```python
from build123d import *

# Parameters (mm, degrees)
F0_R     = 4.8825627193
F0_R_2   = 12.5
F1_DEPTH = 20
F2_R     = 5


with BuildPart() as f1:
    # F0 (on Front) → F1 (new body)
    with BuildSketch(Plane.XZ):
        with BuildLine():
            Line((-24.8438301682, -42.8251363337), (24.8438301682, -42.8251363337))
            Line((24.8438301682, -42.8251363337), (44.8438301682, -20.8251363337))
            Line((44.8438301682, -20.8251363337), (44.8438301682, 42.8251363337))
            Line((44.8438301682, 42.8251363337), (19.4535404444, 42.8251363337))
            Line((19.4535404444, 42.8251363337), (19.4535404444, 22.1680208296))
            ThreePointArc((19.4535404444, 22.1680208296), (17.9890743503, 18.6324869236), (14.4535404444, 17.1680208296))
            Line((14.4535404444, 17.1680208296), (-14.4535404444, 17.1680208296))
            ThreePointArc((-14.4535404444, 17.1680208296), (-17.9890743503, 18.6324869236), (-19.4535404444, 22.1680208296))
            Line((-19.4535404444, 22.1680208296), (-19.4535404444, 42.8251363337))
            Line((-19.4535404444, 42.8251363337), (-44.8438301682, 42.8251363337))
            Line((-44.8438301682, 42.8251363337), (-44.8438301682, -20.8251363337))
            Line((-44.8438301682, -20.8251363337), (-24.8438301682, -42.8251363337))
        make_face()
        with Locations((0, -24.5446097106)):
            Circle(F0_R, mode=Mode.SUBTRACT)
        Circle(F0_R_2, mode=Mode.SUBTRACT)
    extrude(amount=F1_DEPTH)

    # F2
    f2_edges = [f1.edges().sort_by_distance(p)[0] for p in [
        (44.84383, -10, 42.825136),
        (-24.84383, -10, -42.825136),
        (24.84383, -10, -42.825136),
        (44.84383, -10, -20.825136),
        (19.45354, -10, 42.825136),
        (-44.84383, -10, 42.825136),
        (-44.84383, -10, -20.825136),
    ]]
    fillet(f2_edges, radius=F2_R)


solid = f1.part
```
For this review, take the finished solid that the model builds, in its own axes (mm). A direction names the side the tool comes from. Coordinates: 2 decimals unless noted, no trailing zeros. Loops run counter-clockwise (first coordinate to the right, second up) from the corner with the lowest first, then second, coordinate; pieces in that order, holes last.
1. Add section B-B, the plane x = 0. Give the boundary of the cut face in (y, z).
2. For line 1 (Z direction, x = 0, y = -6); line 2 (X direction, y = -1.5, z = 25); line 3 (X direction, y = -18.5, z = -10), list the stretches that pass through material, from the lowest coordinate up.
3. Add section A-A, the plane z = 0. Give the boundary of the cut face in (x, y), then the cut area to 3 significant figures.
4. For faces 5 (the cylindrical face through (-24.63, -10.14, -42.41)), 6 (the cylindrical face through (-17.95, -9.86, 18.594)), list the 3-axis set-ups (+Z, -Z, +X, -X, +Y, -Y) from which the entire face can be reached by the end or side of a thin tool; tool diameter is ignored.
5. Insertion check: P1, Ø10, axis at x = -33, y = -16.5, coming from the -Z side; P2, Ø2, axis at x = 36, y = -17, coming from the -Z side. Each pin has a flat end and moves straight along its axis. Give the tip position at first contact, or say it passes through.
6. Add section C-C, the plane y = -3. Give the boundary of the cut face in (x, z).
7. Mouldability with a two-part tool opening along Z and no side actions: class faces 1 (the cylindrical face through (-0.6, -9.9, -19.7)), 2 (the cylindrical face through (11.923, -9.86, 3.755)), 3 (the flat face through (19.454, -10, 30)), 4 (the cylindrical face through (43.42, -10.14, 41.32)) as +Z half, -Z half, draft (parallel to the pull), parting line (faces both ways), or undercut.
8. Add section D-D, the plane z = 33. Give the boundary of the cut face in (x, y).
Result:
1. outline: (-20, -42.83) - (0, -42.83) - (0, -29.43) - (-20, -29.43) - close; (-20, -19.66) - (0, -19.66) - (0, -12.5) - (-20, -12.5) - close; (-20, 12.5) - (0, 12.5) - (0, 17.17) - (-20, 17.17) - close
2. line 1: z = -42.83 to -29.43, -19.66 to -12.5, 12.5 to 17.17
2. line 2: x = -44.84 to -19.45, 19.45 to 44.84
2. line 3: x = -44.84 to -7.5, 7.5 to 44.84
3. outline: (-44.84, -20) - (-12.5, -20) - (-12.5, 0) - (-44.84, 0) - close; (12.5, -20) - (44.84, -20) - (44.84, 0) - (12.5, 0) - close
3. area: 1,290 mm2
4. face 5: -Z, -X, +Y, -Y
4. face 6: +Z, +Y, -Y
5. P1: stops at z = -39.35
5. P2: stops at z = -31.65
6. outline: (-44.84, -18.89) arc R5 ccw to (-43.54, -22.26) - (-26.33, -41.19) arc R5 ccw to (-22.63, -42.83) - (22.63, -42.83) arc R5 ccw to (26.33, -41.19) - (43.54, -22.26) arc R5 ccw to (44.84, -18.89) - (44.84, 37.83) arc R5 ccw to (39.84, 42.83) - (24.45, 42.83) arc R5 ccw to (19.45, 37.83) - (19.45, 22.17) arc R5 cw to (14.45, 17.17) - (-14.45, 17.17) arc R5 cw to (-19.45, 22.17) - (-19.45, 42.83) - (-39.84, 42.83) arc R5 ccw to (-44.84, 37.83) - close; hole circle Ø25 at (0, 0); hole circle Ø9.77 at (0, -24.54)
7. face 1: undercut
7. face 2: undercut
7. face 3: draft
7. face 4: +Z half
8. outline: (-44.84, -20) - (-19.45, -20) - (-19.45, 0) - (-44.84, 0) - close; (19.45, -20) - (44.84, -20) - (44.84, 0) - (19.45, 0) - close
